Can you work these out from the model? Positions are in its coordinate system, mm. Face numbers are marked on the shaded views. A direction names the side the tool comes from. Coordinates: 2 decimals unless noted, no trailing zeros. Write each loop counter-clockwise with the first axis right and the second up, starting at its lowest first coordinate (ties: lowest second). Pieces come first, ordered by that corner, then holes. Notation, with made-up numbers: (74.25, -4) - (85.25, -4) arc R21 cw to (85.25, 18) - close; hole circle Ø6 at (-18.5, -32.5). An arc over 180 degrees is marked (long way). Use one line per item in the form item = value. Start each with the question number.
(1) If we section it at A-A on z = 12: Please give me the cut outline in (x, y), then the cut area to 3 significant figures.
(2) If I drill on probe 1 along X at (y, z) = (19, 91.5); probe 2 along Z at (x, y) = (-27.5, 15); probe 3 along Y at (x, z) = (28.5, 90), over which ranges is the centre line in solid material (lowest first)? Write a range as from..to.
(3) On a 3-axis mill with a long thin cutter (end or side, diameter ignored), from which of +Z, -Z, +X, -X, +Y, -Y can I reach the whole of each face in a straight line? I mean the marked faces 1, 2, 3, 4 and 5. Say none if no direction works.
(4) For pin 1 Ø19.5 at (y, z) = (-11.5, 85.5) entering from +X; pin 2 Ø3 at (y, z) = (3.5, 62.5) entering from -X; pin 3 Ø10 at (x, z) = (-7, 23.5) entering from -Y, each with a flat end and sliding along its axis, tell me the tip position at first contact or that it passes through.
(5) If we section it at B-B on y = -45: Please give me the cut outline in (x, z), then the cut area to 3 significant figures.
(6) If we section it at C-C on x = 6: Please give me the cut outline in (y, z).
Autodesk Inventor part; units mm, degrees
ref_plane "YZ Plane" through (0, 0, 0) normal (1, 0, 0) x (0, 1, 0)
ref_plane "XZ Plane" through (0, 0, 0) normal (0, 1, 0) x (-1, 0, 0)
ref_plane "XY Plane" through (0, 0, 0) normal (0, 0, 1) x (1, 0, 0)
sketch "Sketch1" plane through (0, 0, 0) normal (0, 0, 1) x (1, 0, 0)
  line L0 (0, 50) -> (43.3013, 25)
  line L1 (43.3013, 25) -> (43.3013, -25)
  line L2 (43.3013, -25) -> (0, -50)
  line L3 (0, -50) -> (-43.3013, -25)
  line L4 (-43.3013, -25) -> (-43.3013, 25)
  line L5 (-43.3013, 25) -> (0, 50)
  line L6 (-43.3013, 0) -> (-41.8013, 0)
  line L7 (-41.8013, 0) -> (-41.8013, 19.6162)
  line L8 (-41.8013, 0) -> (-41.8013, -22.4019)
  line L9 (-41.8013, 24.1299) -> (-0.0035, 48.2659)
  line L10 (-0.0035, 48.2659) -> (41.7978, 24.136)
  line L11 (41.7978, 24.136) -> (41.8013, -24.1299)
  line L12 (41.8013, -24.1299) -> (0.0035, -48.2659)
  line L13 (0.0035, -48.2659) -> (-41.7978, -24.136)
  line L14 (-41.7978, -24.136) -> (-41.8013, 24.1299)
  point P0 (0, 0)
  point P1 (41.8008, -18.0468)
  point P2 (43.3013, -18.0468)
  point P3 (41.8009, -18.3387)
  point P4 (43.3013, -18.3387)
  dimension "d0" = 50
  dimension "d11" = 1.5
  dimension "d12" = 0.004
  dimension "d13" = 1.5004
extrude "Extrusion3" add sketch "Sketch1" along normal blind 150
sketch "Sketch2" plane through (0, 0, 150) normal (0, 0, 1) x (1, 0, 0)
  line L0 (0, 0) -> (0, 52)
  line L1 (0, 52) -> (45.0333, 26)
  line L2 (45.0333, 26) -> (45.0333, -26)
  line L3 (45.0333, -26) -> (0, -52)
  line L4 (0, -52) -> (-45.0333, -26)
  line L5 (-45.0333, -26) -> (-45.0333, 26)
  line L6 (-45.0333, 26) -> (0, 52)
  dimension "d16" = 52
  dimension "d17" = 52
extrude "Extrusion4" add sketch "Sketch2" along normal blind 1.5
sketch "Sketch3" plane through (0, 0, 0) normal (0, 0, -1) x (-1, 0, 0)
  line L0 (45.0333, -26) -> (0, -52)
  line L1 (0, -52) -> (-45.0333, -26)
  line L2 (-45.0333, -26) -> (-45.0333, 26)
  line L3 (-45.0333, 26) -> (0, 52)
  line L4 (0, 52) -> (45.0333, 26)
  line L5 (45.0333, 26) -> (45.0333, -26)
  line L6 (45.0333, -26) -> (0, -52)
  point P0 (0, 0)
  point P1 (0, 0)
  dimension "d20" = 52
extrude "Extrusion5" add sketch "Sketch3" along normal blind 1.5
properties part number "Hexagono"
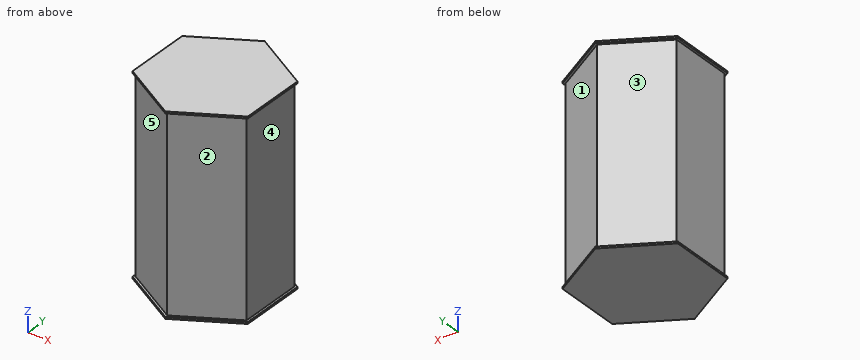
Reported:
q1.outline = (-43.3, -25) - (0, -50) - (43.3, -25) - (43.3, 25) - (0, 50) - (-43.3, 25) - close; hole (-41.8, -24.14) - (0, -48.27) - (41.8, -24.13) - (41.8, 24.14) - (0, 48.27) - (-41.8, 24.13) - (-41.8, 19.62) - (-41.8, 0) - close
q1.area = 443 mm2
q2.probe_1 = -43.3..-41.8, 41.8..43.3
q2.probe_2 = -1.5..0, 150..151.5
q2.probe_3 = -33.55..-31.81, 31.81..33.55
q3.face_1 = +X, +Y
q3.face_2 = +X, -Y
q3.face_3 = -X, +Y
q3.face_4 = +X, +Y, -Y
q3.face_5 = -X, -Y
q4.pin_1 = 43.3
q4.pin_2 = -43.3
q4.pin_3 = -48.85
q5.outline = (-12.12, -1.5) - (12.12, -1.5) - (12.12, 0) - (8.66, 0) - (8.66, 150) - (12.12, 150) - (12.12, 151.5) - (-12.12, 151.5) - (-12.12, 150) - (-8.66, 150) - (-8.66, 0) - (-12.12, 0) - close; hole (-5.65, 0) - (5.66, 0) - (5.66, 150) - (-5.65, 150) - close
q5.area = 974 mm2
q6.outline = (-48.54, -1.5) - (48.54, -1.5) - (48.54, 0) - (46.54, 0) - (46.54, 150) - (48.54, 150) - (48.54, 151.5) - (-48.54, 151.5) - (-48.54, 150) - (-46.54, 150) - (-46.54, 0) - (-48.54, 0) - close; hole (-44.8, 0) - (44.8, 0) - (44.8, 150) - (-44.8, 150) - close
